```python
from build123d import *

# Parameters (mm, degrees)
F0_W      = 45.2956259251
F0_H      = 35.350099206
F1_DEPTH  = 40
F2_DEPTH  = 2900
F3_DEPTH  = 600
F4_DEPTH  = 2850
F5_DEPTH  = 50
F6_DEPTH  = 25
F7_DEPTH  = 10
F8_DEPTH  = 5
F9_DEPTH  = 2
F10_DEPTH = 1
F11_R     = 3
F12_W     = 559.0722560883
F12_H     = 383.7698698044
F13_DEPTH = 40
F14_DEPTH = 40
F15_DEPTH = 25
F16_DEPTH = 30
F17_DEPTH = 400
F18_DEPTH = 60
F19_DEPTH = 40
F20_DEPTH = 250
F21_DEPTH = 50


with BuildPart() as f1:
    # F0 (on Top) → F1 (new body)
    with BuildSketch(Plane.XY):
        with Locations((22.6478129625, -17.675049603)):
            Rectangle(F0_W, F0_H)
    extrude(amount=F1_DEPTH)

    # F2 (add): a face of the model
    f2_faces = [f1.faces().sort_by_distance(p)[0] for p in [
        (0, -17.675049603, 20),
    ]]
    extrude(f2_faces, amount=-F2_DEPTH)

    # F3 (add): a face of the model
    f3_faces = [f1.faces().sort_by_distance(p)[0] for p in [
        (1450, 0, 20),
    ]]
    extrude(f3_faces, amount=-F3_DEPTH)

    # F4 (add): a face of the model
    f4_faces = [f1.faces().sort_by_distance(p)[0] for p in [
        (0, -300, 20),
    ]]
    extrude(f4_faces, amount=-F4_DEPTH)

    # F5 (cut): a face of the model
    f5_faces = [f1.faces().sort_by_distance(p)[0] for p in [
        (2900, -300, 20),
    ]]
    extrude(f5_faces, amount=-F5_DEPTH, mode=Mode.SUBTRACT)

    # F6 (cut): a face of the model
    f6_faces = [f1.faces().sort_by_distance(p)[0] for p in [
        (2850, -300, 20),
    ]]
    extrude(f6_faces, amount=-F6_DEPTH, mode=Mode.SUBTRACT)

    # F7 (add): a face of the model
    f7_faces = [f1.faces().sort_by_distance(p)[0] for p in [
        (2825, -300, 20),
    ]]
    extrude(f7_faces, amount=F7_DEPTH)

    # F8 (cut): a face of the model
    f8_faces = [f1.faces().sort_by_distance(p)[0] for p in [
        (2835, -300, 20),
    ]]
    extrude(f8_faces, amount=-F8_DEPTH, mode=Mode.SUBTRACT)

    # F9 (add): a face of the model
    f9_faces = [f1.faces().sort_by_distance(p)[0] for p in [
        (2830, -300, 20),
    ]]
    extrude(f9_faces, amount=F9_DEPTH)

    # F10 (cut): a face of the model
    f10_faces = [f1.faces().sort_by_distance(p)[0] for p in [
        (2832, -300, 20),
    ]]
    extrude(f10_faces, amount=-F10_DEPTH, mode=Mode.SUBTRACT)

    # F11
    f11_edges = [f1.edges().sort_by_distance(p)[0] for p in [
        (1415.5, -600, 40),
        (0, -300, 40),
        (0, -600, 20),
        (1415.5, -600, 0),
        (0, -300, 0),
    ]]
    fillet(f11_edges, radius=F11_R)

    # F12 (on face) → F13 (cut)
    with BuildSketch(Plane.XY.offset(40)):
        with Locations((2405.6543111801, -302.7966022491)):
            Rectangle(F12_W, F12_H)
    extrude(amount=-F13_DEPTH, mode=Mode.SUBTRACT)

    # F14 (cut): a face of the model
    f14_faces = [f1.faces().sort_by_distance(p)[0] for p in [
        (2405.6543111801, -494.6815371513, 20),
    ]]
    extrude(f14_faces, amount=-F14_DEPTH, mode=Mode.SUBTRACT)

    # F15 (cut): a face of the model
    f15_faces = [f1.faces().sort_by_distance(p)[0] for p in [
        (2405.6543111801, -110.911667347, 20),
    ]]
    extrude(f15_faces, amount=-F15_DEPTH, mode=Mode.SUBTRACT)

    # F16 (cut): a face of the model
    f16_faces = [f1.faces().sort_by_distance(p)[0] for p in [
        (2405.6543111801, -85.911667347, 20),
    ]]
    extrude(f16_faces, amount=-F16_DEPTH, mode=Mode.SUBTRACT)

    # F17 (cut): a face of the model
    f17_faces = [f1.faces().sort_by_distance(p)[0] for p in [
        (2126.118183136, -295.2966022491, 20),
    ]]
    extrude(f17_faces, amount=-F17_DEPTH, mode=Mode.SUBTRACT)

    # F18 (add): a face of the model
    f18_faces = [f1.faces().sort_by_distance(p)[0] for p in [
        (1726.118183136, -295.2966022491, 20),
    ]]
    extrude(f18_faces, amount=F18_DEPTH)

    # F19 (add): a face of the model
    f19_faces = [f1.faces().sort_by_distance(p)[0] for p in [
        (1786.118183136, -295.2966022491, 20),
    ]]
    extrude(f19_faces, amount=F19_DEPTH)

    # F20 (add): a face of the model
    f20_faces = [f1.faces().sort_by_distance(p)[0] for p in [
        (2685.1904392242, -295.2966022491, 20),
    ]]
    extrude(f20_faces, amount=F20_DEPTH)

    # F21 (add): a face of the model
    f21_faces = [f1.faces().sort_by_distance(p)[0] for p in [
        (2435.1904392242, -295.2966022491, 20),
    ]]
    extrude(f21_faces, amount=F21_DEPTH)


solid = f1.part
```
CAD build for the part. Positions are in the model's coordinates, mm. Coordinates: 2 decimals unless noted, no trailing zeros. Order: outer loops, then holes, each group sorted by start corner. A loop starts at its lowest first (then second) coordinate and runs counter-clockwise, first axis right, second up. Notation, with made-up numbers: (70.25, 26.25) - (111.25, 26.25) arc R23 cw to (111.25, 37.25) - close; hole circle Ø4 at (47.25, 5). An arc over 180 degrees is marked (long way). Use a Markdown table: item, result. Add a question column.
(1) Saw through at A-A (x = 2173). Give the cut face in (y, z), then the cut area to 3 significant figures.
(2) Saw through at C-C (z = 13.5). Give the cut face in (x, y), then the cut area to 3 significant figures.
(3) Drill centre lines: line 1 along X through (y, z) = (-252.5, 5); line 2 along Y through (x, z) = (2243, 29.5). Where is each one in solid material? Low to high. Write a range as [from, to].
(4) Flat gauge pin, fed straight in: pin 1 (10 mm diameter, centred on x = 1030.5, z = 16, fed in from +Y). Where does the tip first touch, or does it go through?
(5) Saw through at B-B (y = -496). Give the cut face in (x, z).
Solved:
| question | item | result |
|---|---|---|
| 1 | outline | (-600, 3) arc R3 ccw to (-597, 0) - (-534.68, 0) - (-534.68, 40) - (-597, 40) arc R3 ccw to (-600, 37) - close; (-55.91, 0) - (0, 0) - (0, 40) - (-55.91, 40) - close |
| 1 | area | 4,850 mm² |
| 2 | outline | (0, -597) arc R3 ccw to (3, -600) - (2831, -600) - (2831, 0) - (0, 0) - close; hole (1826.12, -534.68) - (2385.19, -534.68) - (2385.19, -55.91) - (1826.12, -55.91) - close |
| 2 | area | 1,430,000 mm² |
| 3 | line 1 | x = [0, 1826.12], [2385.19, 2831] |
| 3 | line 2 | y = [-600, -534.68], [-55.91, 0] |
| 4 | pin 1 | stops at y = 0 |
| 5 | outline | (0, 3) arc R3 ccw to (3, 0) - (1826.12, 0) - (1826.12, 40) - (3, 40) arc R3 ccw to (0, 37) - close; (2385.19, 0) - (2831, 0) - (2831, 40) - (2385.19, 40) - close |
